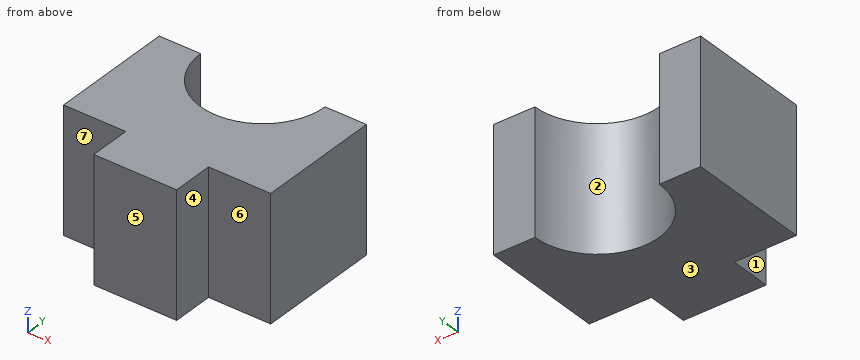
```python
from build123d import *

# Parameters (mm, degrees)
CROQUIS1_W              = 25
CROQUIS1_H              = 15
SALIENTE_EXTRUIR1_DEPTH = 20
CROQUIS2_W              = 7.5
CROQUIS2_H              = 5
CORTAR_EXTRUIR1_DEPTH   = 20
CROQUIS3_R              = 7.5
CORTAR_EXTRUIR2_DEPTH   = 20


with BuildPart() as part:
    # Croquis1 → Saliente-Extruir1 (new body)
    with BuildSketch(Plane(origin=(0, 0, 0), x_dir=(1, 0, 0), z_dir=(0, 1, 0))):
        with Locations((12.5, -7.5)):
            Rectangle(CROQUIS1_W, CROQUIS1_H)
    extrude(amount=SALIENTE_EXTRUIR1_DEPTH)

    # Croquis2 → Cortar-Extruir1 (cut)
    with BuildSketch(Plane.XY.offset(15)):
        with Locations((21.25, 2.5)):
            Rectangle(CROQUIS2_W, CROQUIS2_H)
        with Locations((3.75, 2.5)):
            Rectangle(CROQUIS2_W, CROQUIS2_H)
    extrude(amount=-CORTAR_EXTRUIR1_DEPTH, mode=Mode.SUBTRACT)

    # Croquis3 → Cortar-Extruir2 (cut)
    with BuildSketch(Plane.XY.offset(15)):
        with Locations((12.5, 20)):
            Circle(CROQUIS3_R)
    extrude(amount=-CORTAR_EXTRUIR2_DEPTH, mode=Mode.SUBTRACT)


solid = part.part
```
Design review of the part built by this model. Coordinates are the model's own, in mm. Face numbers are marked on the shaded views. A direction names the side the tool comes from. Coordinates: 2 decimals unless noted, no trailing zeros. Order: outer loops, then holes, each group sorted by start corner. A loop starts at its lowest first (then second) coordinate and runs counter-clockwise, first axis right, second up. Notation, with made-up numbers: (-16.5, 84.5) -> (21.5, 84.5) arc R30 cw to (21.5, 109.5) -> close; hole circle Ø8 at (-32, 10.5). An arc over 180 degrees is marked (long way). One line per item, written item: value. Start each with the question number.
Q1. Take a section at B-B, the plane z = 4. State the section outline as (x, y) points, then the cut area to 3 significant figures.
Q2. Take a section at A-A, the plane y = 13.75. State the section outline as (x, z) points.
Q3. For probe 1 along Y at (x, z) = (1.75, 11.75); probe 2 along X at (y, z) = (4, 1.25); probe 3 along X at (y, z) = (13.75, 7.75), list the stretches that pass through material, from the lowest coordinate up.
Q4. Take a section at C-C, the plane y = 4. State the section outline as (x, z) points, then the cut area to 3 significant figures.
Q5. Take a section at D-D, the plane x = 12.5. State the section outline as (y, z) points.
Q6. Tool access review of the marked faces 5, 6 and 7: name each direction out of +Z, -Z, +X, -X, +Y, -Y from which nothing blocks a thin tool from reaching the whole face with its end or side.
Q7. Insertion check: pin 1 Ø4 at (x, z) = (4.5, 5.5) entering from -Y; pin 2 Ø4 at (y, z) = (2.5, 11) entering from -X; pin 3 Ø2.5 at (y, z) = (3, 10) entering from +X. Each pin has a flat end and moves straight along its axis. Give the tip position at first contact, or say it passes through.
Q8. Mouldability with a two-part tool opening along X and no side actions: class the marked faces 1, 2, 3 and 4 as pulls with the +X half, pulls with the -X half, needs draft (parallel to the pull), parting line crosses it, or undercut.
Values follow:
1. outline: (0, 5) -> (7.5, 5) -> (7.5, 0) -> (17.5, 0) -> (17.5, 5) -> (25, 5) -> (25, 20) -> (20, 20) arc R7.5 cw to (5, 20) -> (0, 20) -> close
1. area: 337 mm2
2. outline: (0, 0) -> (8.35, 0) -> (8.35, 15) -> (0, 15) -> close; (16.65, 0) -> (25, 0) -> (25, 15) -> (16.65, 15) -> close
3. probe 1: y = 5 to 20
3. probe 2: x = 7.5 to 17.5
3. probe 3: x = 0 to 8.35, 16.65 to 25
4. outline: (7.5, 0) -> (17.5, 0) -> (17.5, 15) -> (7.5, 15) -> close
4. area: 150 mm2
5. outline: (0, 0) -> (12.5, 0) -> (12.5, 15) -> (0, 15) -> close
6. face 5: +Z, -Z, +X, -X, -Y
6. face 6: +Z, -Z, +X, -Y
6. face 7: +Z, -Z, -X, -Y
7. pin 1: stops at y = 5
7. pin 2: stops at x = 7.5
7. pin 3: stops at x = 17.5
8. face 1: pulls with the -X half
8. face 2: undercut
8. face 3: needs draft
8. face 4: pulls with the +X half
